Can you work these out from the model? Positions are in its coordinate system, mm. A direction names the side the tool comes from. Give positions to 0.01 mm unless a question says otherwise; leave off trailing zeros. Order: outer loops, then holes, each group sorted by start corner. A loop starts at its lowest first (then second) coordinate and runs counter-clockwise, first axis right, second up.
Item 1: I want a section at B-B, the plane z = -65. Write out the boundary of the cut face in (x, y), then the cut area to 3 significant figures.
Item 2: I want a section at A-A, the plane x = -59.5. Write out the boundary of the cut face in (y, z).
Item 3: If we mould it in two halves opening along Z, with no side actions, what happens to faces 1 (the flat face through (-46, 0, -26)), 2 (the flat face through (21.37, -12.52, 56.53)), 3 (the flat face through (33.755, -12.522, -36.567))? For each: +Z half, -Z half, draft (parallel to the pull), parting line (faces both ways), or undercut.
Item 4: I want a section at D-D, the plane x = 105. Write out the boundary of the cut face in (y, z), then the cut area to 3 significant figures.
Item 5: I want a section at C-C, the plane y = -21.25. Write out the boundary of the cut face in (x, z).
Item 6: Which directions (+Z, -Z, +X, -X, +Y, -Y) give clear straight access to the entire face, cutting with the end or side of a thin tool? Please do faces 4 (the flat face through (14.79, -12.522, 47.516)), 5 (the flat face through (38.27, -12.52, -46.77)).
Item 7: If I drill on line 1 along X through (y, z) = (-1.25, -16); line 2 along X through (y, z) = (-16.25, -58.5); line 3 along Z through (x, y) = (63, -16.75), over which ranges is the centre line in solid material (lowest first)?
Item 8: I'm going to push flat-ended pins straight in: pin 1 Ø12 at (x, y) = (26.5, -4) entering from -Z; pin 2 Ø4 at (x, y) = (32.5, -15) entering from -Z; pin 3 Ø5 at (x, y) = (-29.5, -8.5) entering from -Z. Where does each tip first touch, or does it pass through?
```python
from build123d import *

# Parameters (mm, degrees)
F1_DEPTH = 25.4


with BuildPart() as f1:
    # F0 (on Front) → F1 (new body)
    with BuildSketch(Plane.XZ):
        Polygon((-39.975051, -114.025376), (118.736398, 22.393278), (-78.761347, 91.632098), align=None)
        Polygon((-65.698497, 74.72723), (97.564928, 19.532953), (-31.866431, -94.260182), align=None, mode=Mode.SUBTRACT)
    extrude(amount=F1_DEPTH)


solid = f1.part
```
Results list:
1. outline: (-49.22, -25.4) - (-37.72, -25.4) - (-37.72, 0) - (-49.22, 0) - close; (1.41, -25.4) - (17.06, -25.4) - (17.06, 0) - (1.41, 0) - close
1. area: 689 mm2
2. outline: (-25.4, -10.5) - (0, -10.5) - (0, 43.77) - (-25.4, 43.77) - close; (-25.4, 72.63) - (0, 72.63) - (0, 84.88) - (-25.4, 84.88) - close
3. face 1: draft
3. face 2: +Z half
3. face 3: undercut
4. outline: (-25.4, 10.59) - (0, 10.59) - (0, 27.21) - (-25.4, 27.21) - close
4. area: 422 mm2
5. outline: (-78.76, 91.63) - (-39.98, -114.03) - (118.74, 22.39) - close; hole (-65.7, 74.73) - (-31.87, -94.26) - (97.56, 19.53) - close
6. face 4: +Y, -Y
6. face 5: -Z, +X, +Y, -Y
7. line 1: x = -58.46 to -47.53, 57.15 to 74.07
7. line 2: x = -50.45 to -39.03, 8.81 to 24.62
7. line 3: z = -25.51 to -10.86, 31.22 to 41.93
8. pin 1: stops at z = -62.04
8. pin 2: stops at z = -53.45
8. pin 3: stops at z = -107.17
